Design review of the part built by this model. Coordinates are the model's own, in mm. Face numbers are marked on the shaded views. A direction names the side the tool comes from. Round coordinates to 2 decimals unless told otherwise and drop trailing zeros. Write each loop counter-clockwise with the first axis right and the second up, starting at its lowest first coordinate (ties: lowest second). Pieces come first, ordered by that corner, then holes. Notation, with made-up numbers: (33, -10) -> (49, -10) arc R22 ccw to (49, 13) -> close; hole circle Ø7 at (-3.75, -18.75). An arc over 180 degrees is marked (long way). Write item = value, one per line. Start each with the question number.
Item 1: Add section D-D, the plane x = 11.5. State the section outline as (y, z) points.
Item 2: Machinability: for the marked faces 5, 6, 7, 8 and 9, which of the approach directions +Z, -Z, +X, -X, +Y, -Y give a long, thin tool a straight path to every point of the face, cutting with its end or side? Answer none if there is none.
Item 3: Mouldability with a two-part tool opening along Y and no side actions: class the marked faces 1, 2, 3 and 4 as released by +Y, released by -Y, zero draft, split by the parting line, or undercut.
Item 4: Add section A-A, the plane z = -2. State the section outline as (x, y) points.
Item 5: Add section B-B, the plane x = -16. State the section outline as (y, z) points, then the cut area to 3 significant figures.
Item 6: Add section C-C, the plane y = 6. State the section outline as (x, z) points, then the cut area to 3 significant figures.
Item 7: To check wall thickness, follow L1, parallel to Y at x = -13.5, z = -2; L2, parallel to Y at x = -6, z = -7.5; L3, parallel to X at y = 7.5, z = 1.5. State the ranges of each line that lie inside material, in increasing order.
Item 8: For pin 1 Ø4 at (x, z) = (-8, -3) entering from -Y; pin 2 Ø10 at (y, z) = (-8.5, -1.5) entering from -X; pin 3 Ø1.5 at (x, y) = (-24, 0.5) entering from +Z; pin 4 Ø9.5 at (x, z) = (-18.5, -3.5) entering from +Y, all flat-tipped, find the tip position at first contact; note any pin that passes through.
from build123d import *

# Parameters (mm, degrees)
F1_DEPTH  = 11.25
F4_DEPTH  = 12.5
F8_DEPTH  = 25
F9_DEPTH  = 5
F10_DEPTH = 5


with BuildPart() as f1:
    # F0 (on Top) → F1 (new body)
    with BuildSketch(Plane.XY):
        with BuildLine():
            Line((-22, 0), (0, 0))
            Line((0, 0), (17, 0))
            ThreePointArc((17, 0), (24.313496, 5.837842), (20.24165, 14.263261))
            Line((20.24165, 14.263261), (4.545653, 21.786397))
            ThreePointArc((4.545653, 21.786397), (4.091542, 21.811059), (3.752999, 21.507393))
            Line((3.752999, 21.507393), (3.186098, 20.324631))
            ThreePointArc((3.186098, 20.324631), (3.161436, 19.87052), (3.465103, 19.531977))
            Line((3.465103, 19.531977), (19.1611, 12.008841))
            ThreePointArc((19.1611, 12.008841), (21.875664, 6.391894), (17, 2.5))
            Line((17, 2.5), (-22, 2.5))
            ThreePointArc((-22, 2.5), (-29.5, -5), (-22, -12.5))
            Line((-22, -12.5), (-10.142284, -12.5))
            ThreePointArc((-10.142284, -12.5), (-10.003912, -12.483664), (-9.873148, -12.435554))
            Line((-9.873148, -12.435554), (-4.978775, -9.949009))
            ThreePointArc((-4.978775, -9.949009), (-4.678281, -9.588354), (-4.73332, -9.122157))
            Line((-4.73332, -9.122157), (-5.372774, -8.014591))
            ThreePointArc((-5.372774, -8.014591), (-5.733575, -7.737739), (-6.184464, -7.797099))
            Line((-6.184464, -7.797099), (-9.862116, -9.920392))
            ThreePointArc((-9.862116, -9.920392), (-10.005425, -9.979753), (-10.159215, -10))
            Line((-10.159215, -10), (-22, -10))
            ThreePointArc((-22, -10), (-27, -5), (-22, 0))
        make_face()
    extrude(amount=F1_DEPTH)

    # F3 (on offset) → F4 (cut)
    with BuildSketch(Plane.XZ.offset(5)):
        Polygon((27.003047, 6.75), (27.003047, 15.756967), (-27, 11.25), align=None)
    extrude(amount=-F4_DEPTH, mode=Mode.SUBTRACT)

    # F6 (on offset) → F8 (cut)
    with BuildSketch(Plane.XZ.offset(-7.5)):
        with BuildLine():
            Line((22, 7.166897), (24.5, 6.958576))
            Line((24.5, 6.958576), (25.517887, 14.069991))
            Line((25.517887, 14.069991), (1.366809, 12.402037))
            Line((1.366809, 12.402037), (3.064071, 5))
            Line((3.064071, 5), (3.064071, 2.323721))
            ThreePointArc((3.064071, 2.323721), (3.825408, 4.320816), (5.722997, 5.304269))
            Line((5.722997, 5.304269), (22, 7.166897))
        make_face()
    extrude(amount=-F8_DEPTH, mode=Mode.SUBTRACT)

    # F7 (on face) → F9 (cut)
    with BuildSketch(Plane(origin=(2.996136, -5.897423, 0), x_dir=(0.891541, 0.45294, 0), z_dir=(0.45294, -0.891541, 0))):
        with BuildLine():
            Line((-7.304974, 12.209089), (-10.371014, 11.25))
            Line((-10.371014, 11.25), (-9.32518, 11.25))
            Line((-9.32518, 11.25), (-8.945085, 11.25))
            Line((-8.945085, 11.25), (-8.945085, 11.174948))
            ThreePointArc((-8.945085, 11.174948), (-8.494489, 10.806734), (-8.32518, 10.25))
            Line((-8.32518, 10.25), (-8.32518, 10.173095))
            Line((-8.32518, 10.173095), (-7.304974, 10.173095))
            Line((-7.304974, 10.173095), (-7.304974, 12.209089))
        make_face()
    extrude(amount=-F9_DEPTH, mode=Mode.SUBTRACT)

    # F7 (on face) → F10 (cut)
    with BuildSketch(Plane(origin=(2.996136, -5.897423, 0), x_dir=(0.891541, 0.45294, 0), z_dir=(0.45294, -0.891541, 0))):
        with BuildLine():
            Line((-7.304974, 12.209089), (-10.371014, 11.25))
            Line((-10.371014, 11.25), (-9.32518, 11.25))
            Line((-9.32518, 11.25), (-8.945085, 11.25))
            Line((-8.945085, 11.25), (-8.945085, 11.174948))
            ThreePointArc((-8.945085, 11.174948), (-8.494489, 10.806734), (-8.32518, 10.25))
            Line((-8.32518, 10.25), (-8.32518, 10.173095))
            Line((-8.32518, 10.173095), (-7.304974, 10.173095))
            Line((-7.304974, 10.173095), (-7.304974, 12.209089))
        make_face()
        with BuildLine():
            Line((-8.945085, 11.25), (-9.32518, 11.25))
            ThreePointArc((-9.32518, 11.25), (-9.131463, 11.231057), (-8.945085, 11.174948))
            Line((-8.945085, 11.174948), (-8.945085, 11.25))
        make_face()
    extrude(amount=-F10_DEPTH, mode=Mode.SUBTRACT)

    # F11: F1 across plane


with BuildPart() as f1_1:
    add(f1.part)
    add(f1.part.mirror(Plane.XY))


solid = f1_1.part
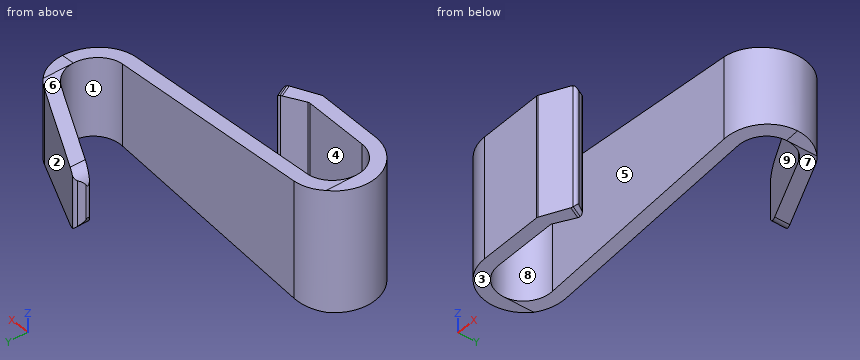
Result set:
q1.outline = (0, -8.04) -> (2.5, -8.04) -> (2.5, 8.04) -> (0, 8.04) -> close; (15.68, -5.97) -> (18.45, -5.97) -> (18.45, 5.97) -> (15.68, 5.97) -> close
q2.face_5 = +Z, -Z, +X
q2.face_6 = +Z, -X, +Y
q2.face_7 = -Z, -X, +Y
q2.face_8 = +Z, -Z
q2.face_9 = +Z, -Z, -X
q3.face_1 = undercut
q3.face_2 = released by +Y
q3.face_3 = zero draft
q3.face_4 = undercut
q4.outline = (-22, -12.5) -> (-10.14, -12.5) arc R0.59 ccw to (-9.87, -12.44) -> (-4.98, -9.95) arc R0.59 ccw to (-4.73, -9.12) -> (-5.37, -8.01) arc R0.59 ccw to (-6.18, -7.8) -> (-9.86, -9.92) arc R0.59 cw to (-10.16, -10) -> (-22, -10) arc R5 cw to (-22, 0) -> (17, 0) arc R7.5 ccw to (20.24, 14.26) -> (4.55, 21.79) arc R0.59 ccw to (3.75, 21.51) -> (3.19, 20.32) arc R0.59 ccw to (3.47, 19.53) -> (19.16, 12.01) arc R5 cw to (17, 2.5) -> (-22, 2.5) arc R7.5 ccw to start
q5.outline = (-12.5, -11.25) -> (-10, -11.25) -> (-10, 11.25) -> (-12.5, 11.25) -> close; (0, -10.33) -> (2.5, -10.33) -> (2.5, 10.33) -> (0, 10.33) -> close
q5.area = 108 mm²
q6.outline = (21.77, -7.19) -> (24.35, -6.97) -> (24.35, 6.97) -> (21.77, 7.19) -> close
q6.area = 36.5 mm²
q7.L1 = -12.5 to -10, 0 to 2.5
q7.L2 = -10.47 to -7.73, 0 to 2.5
q7.L3 = 22 to 24.5
q8.pin_1 = -12.48
q8.pin_2 = -29.5
q8.pin_3 = 11.06
q8.pin_4 = 2.5
